Autodesk Inventor part; units mm, degrees
ref_plane "YZ Plane" through (0, 0, 0) normal (1, 0, 0) x (0, 1, 0)
ref_plane "XZ Plane" through (0, 0, 0) normal (0, 1, 0) x (-1, 0, 0)
ref_plane "XY Plane" through (0, 0, 0) normal (0, 0, 1) x (1, 0, 0)
sketch "Szkic1" plane through (0, 0, 0) normal (0, 0, 1) x (1, 0, 0)
  circle A0 centre (0, 0) radius 15
  dimension "d0" = 30
extrude "Wyciągnięcie proste1" add sketch "Szkic1" along normal mid plane 75
sketch "Szkic2" plane through (0, 0, 0) normal (0, 1, 0) x (-1, 0, 0)
  circle A0 centre (0, 0) radius 7.5
  dimension "d3" = 15
extrude "Wyciągnięcie proste2" cut sketch "Szkic2" along normal mid plane 35
sketch "Szkic3" plane through (0, 0, 37.5) normal (0, 0, 1) x (1, 0, 0)
  circle A0 centre (0, 0) radius 14
  circle A1 centre (0, 0) radius 15
  dimension "d6" = 28
  dimension "d7" = 30
extrude "Wyciągnięcie proste3" cut sketch "Szkic3" against normal blind 15
sketch "Szkic4" plane through (0, 0, -37.5) normal (0, 0, -1) x (-1, 0, 0)
  circle A0 centre (0, 0) radius 14
  circle A1 centre (0, 0) radius 15
  dimension "d10" = 28
  dimension "d11" = 30
extrude "Wyciągnięcie proste4" cut sketch "Szkic4" against normal blind 15
sketch "Szkic6" plane through (0, 0, 0) normal (1, 0, 0) x (0, 1, 0)
  circle A0 centre (0, 0) radius 1.5
  circle A1 centre (0, -30) radius 1.5
  circle A2 centre (0, 30) radius 1.5
  dimension "d18" = 3
  dimension "d19" = 3
  dimension "d20" = 3
extrude "Wyciągnięcie proste6" cut sketch "Szkic6" against normal blind 30
properties part number "srodek" material "Aluminium 6061"
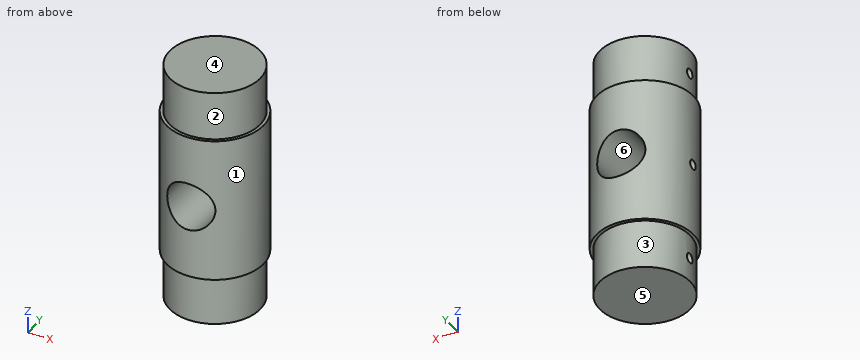
Design review of the part built by this model. Coordinates are the model's own, in mm. Face numbers are marked on the shaded views. A direction names the side the tool comes from. Round coordinates to 2 decimals unless told otherwise and drop trailing zeros. Write each loop counter-clockwise with the first axis right and the second up, starting at its lowest first coordinate (ties: lowest second). Pieces come first, ordered by that corner, then holes.
Item 1: We need section C-C on x = -13. Write out the cut boundary in (y, z), and give its area (3 significant figures).
Item 2: We need section A-A on x = -5. Write out the cut boundary in (y, z), and give its area (3 significant figures).
Item 3: For probe 1 along Z at (x, y) = (-10.5, 0); probe 2 along Z at (x, y) = (-6, 0); probe 3 along Z at (x, y) = (0, -3.75), list the stretches that pass through material, from the lowest coordinate up.
Item 4: For the marked faces 1, 2 and 3, list the 3-axis set-ups (+Z, -Z, +X, -X, +Y, -Y) from which the entire face can be reached by the end or side of a thin tool; tool diameter is ignored.
Item 5: The part is to be moulded in two halves that separate along Z. For the marked faces 4, 5 and 6, say which applies: +Z half, -Z half, draft (parallel to the pull), parting line (faces both ways), or undercut.
Item 6: Clearance check with flat-ended pins moving along their axes: pin 1 Ø3.5 at (y, z) = (0, 30) entering from +X; pin 2 Ø0.9 at (y, z) = (0.5, -29.5) entering from -X; pin 3 Ø2 at (y, z) = (9.5, -5) entering from -X; pin 4 Ø12 at (y, z) = (-3, -17) entering from -X. State where each tip first meets the part, or that it passes through.
Item 7: We need section B-B on y = 4. Write out the cut boundary in (x, z).
Item 8: We need section D-D on y = 0. Write out the cut boundary in (x, z), and give its area (3 significant figures).
Returned:
1. outline: (-7.48, -22.5) - (-5.2, -22.5) - (-5.2, -37.5) - (5.2, -37.5) - (5.2, -22.5) - (7.48, -22.5) - (7.48, 22.5) - (5.2, 22.5) - (5.2, 37.5) - (-5.2, 37.5) - (-5.2, 22.5) - (-7.48, 22.5) - close; hole circle Ø3 at (0, -30); hole circle Ø3 at (0, 0); hole circle Ø3 at (0, 30)
1. area: 964 mm2
2. outline: (-14.14, -22.5) - (-13.08, -22.5) - (-13.08, -37.5) - (13.08, -37.5) - (13.08, -22.5) - (14.14, -22.5) - (14.14, -5.59) - (-14.14, -5.59) - close; (-14.14, 5.59) - (14.14, 5.59) - (14.14, 22.5) - (13.08, 22.5) - (13.08, 37.5) - (-13.08, 37.5) - (-13.08, 22.5) - (-14.14, 22.5) - close; hole circle Ø3 at (0, -30); hole circle Ø3 at (0, 30)
2. area: 1,730 mm2
3. probe 1: z = -37.5 to -31.5, -28.5 to -1.5, 1.5 to 28.5, 31.5 to 37.5
3. probe 2: z = -37.5 to -31.5, -28.5 to -4.5, 4.5 to 28.5, 31.5 to 37.5
3. probe 3: z = -37.5 to -7.5, 7.5 to 37.5
4. face 1: +Z, -Z
4. face 2: +Z
4. face 3: -Z
5. face 4: +Z half
5. face 5: -Z half
5. face 6: undercut
6. pin 1: stops at x = 14
6. pin 2: stops at x = 0
6. pin 3: stops at x = -12.36
6. pin 4: stops at x = -15
7. outline: (-14.46, -22.5) - (-13.42, -22.5) - (-13.42, -37.5) - (13.42, -37.5) - (13.42, -22.5) - (14.46, -22.5) - (14.46, 22.5) - (13.42, 22.5) - (13.42, 37.5) - (-13.42, 37.5) - (-13.42, 22.5) - (-14.46, 22.5) - close; hole circle Ø15 at (0, 0)
8. outline: (-15, -22.5) - (-14, -22.5) - (-14, -28.5) - (0, -28.5) - (0, -31.5) - (-14, -31.5) - (-14, -37.5) - (14, -37.5) - (14, -22.5) - (15, -22.5) - (15, 22.5) - (14, 22.5) - (14, 37.5) - (-14, 37.5) - (-14, 31.5) - (0, 31.5) - (0, 28.5) - (-14, 28.5) - (-14, 22.5) - (-15, 22.5) - (-15, 1.5) - (-7.35, 1.5) arc R7.5 cw (long way) to (-7.35, -1.5) - (-15, -1.5) - close
8. area: 1,910 mm2
